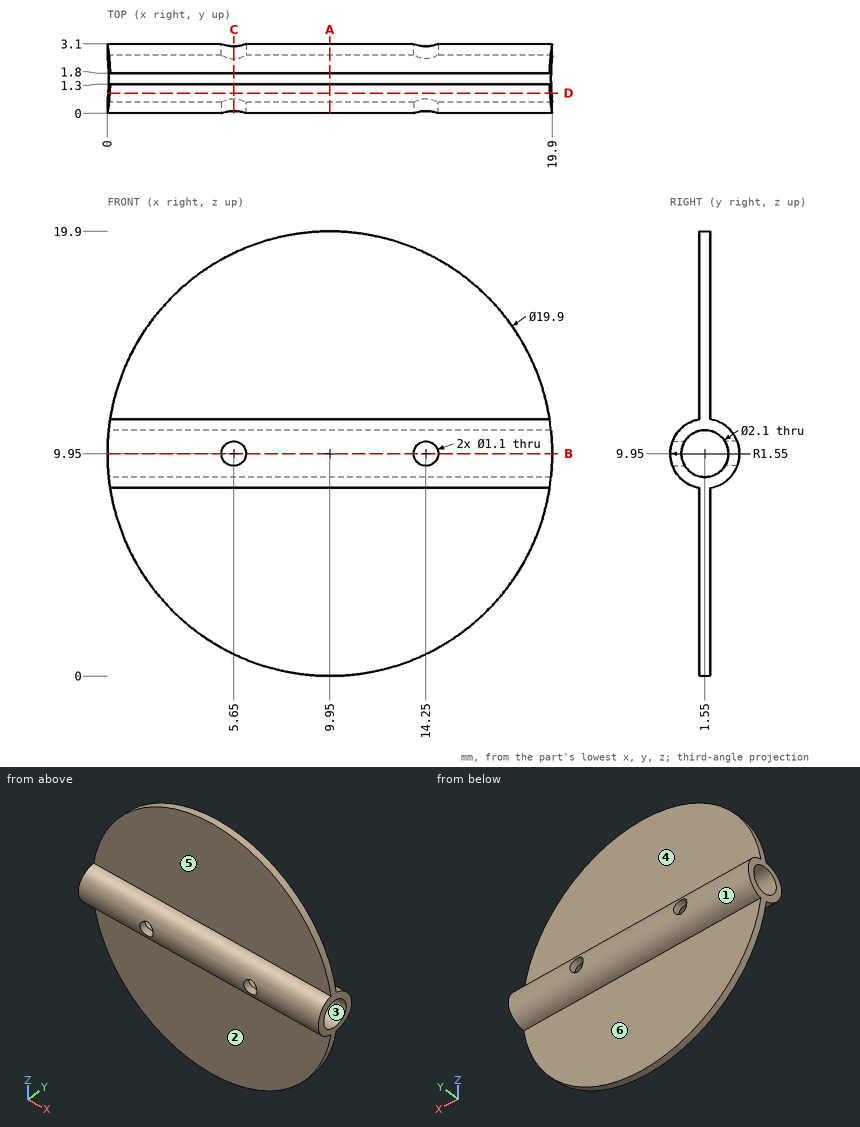
Here's the drawing with two shaded views (mm, measured from the low corner). I have some questions. A direction names the side the tool comes from. Coordinates: 2 decimals unless noted, no trailing zeros. Write each loop counter-clockwise with the first axis right and the second up, starting at its lowest first coordinate (ties: lowest second). Pieces come first, ordered by that corner, then holes. Notation, with made-up numbers: (81, 0) - (129, 0) arc R6 ccw to (129, 9) - close; hole circle Ø11 at (21.25, -17). An arc over 180 degrees is marked (long way). Return JSON: item names as keys, results as strings.
Q1. If we section it at A-A (x = 9.95): Please give me the cut outline in (y, z).
Computed values:
{"outline": "(1.3, 0) - (1.8, 0) - (1.8, 8.42) arc R1.55 ccw to (1.8, 11.48) - (1.8, 19.9) - (1.3, 19.9) - (1.3, 11.48) arc R1.55 ccw to (1.3, 8.42) - close; hole circle Ø2.1 at (1.55, 9.95)"}
Q2. If we section it at B-B (z = 9.95): Please give me the cut outline in (x, y).
Computed values:
{"outline": "(0, 0) - (5.1, 0) - (5.1, 0.5) - (0, 0.5) - close; (0, 2.6) - (5.1, 2.6) - (5.1, 3.1) - (0, 3.1) - close; (6.2, 0) - (13.7, 0) - (13.7, 0.5) - (6.2, 0.5) - close; (6.2, 2.6) - (13.7, 2.6) - (13.7, 3.1) - (6.2, 3.1) - close; (14.8, 0) - (19.9, 0) - (19.9, 0.5) - (14.8, 0.5) - close; (14.8, 2.6) - (19.9, 2.6) - (19.9, 3.1) - (14.8, 3.1) - close"}
Q3. On a 3-axis mill with a long thin cutter (end or side, diameter ignored), from which of +Z, -Z, +X, -X, +Y, -Y can I reach the whole of each face in a straight line? I mean the marked faces 4, 5 and 6. Say none if no direction works.
Computed values:
{"face 4": "+Z, +X, -X, +Y", "face 5": "+Z, +X, -X, -Y", "face 6": "-Z, +X, -X, +Y"}
Q4. Thinking about a two-plate mould opening in Y: for the marked faces 1, 2 and 3, which applies, +Y half, -Y half, draft (parallel to the pull), parting line (faces both ways), or undercut?
Computed values:
{"face 1": "+Y half", "face 2": "-Y half", "face 3": "undercut"}
Q5. If we section it at D-D (y = 0.9): Please give me the cut outline in (x, z).
Computed values:
{"outline": "(0.03, 9.13) arc R9.95 ccw to (0.1, 8.54) - (19.8, 8.54) arc R9.95 ccw to (19.87, 9.13) - close; (0.03, 10.77) - (19.87, 10.77) arc R9.95 ccw to (19.8, 11.36) - (0.1, 11.36) arc R9.95 ccw to start"}
Q6. Please list where these lines run through material, in increasing order: L1, parallel to Y at x = 4.5, z = 15.75; L2, parallel to Z at x = 12, y = 0.85; L3, parallel to Z at x = 4.25, y = 1.9. Write a range as from..to.
Computed values:
{"L1": "y = 1.3..1.8", "L2": "z = 8.57..9.17, 10.73..11.33", "L3": "z = 8.44..8.96, 10.94..11.46"}
Q7. I'm going to push flat-ended pins straight in: pin 1 Ø4 at (x, z) = (10, 4.5) entering from -Y; pin 2 Ø4 at (x, z) = (12, 4.5) entering from +Y; pin 3 Ø6 at (x, z) = (5, 6) entering from -Y. Where does each tip first touch, or does it pass through?
Computed values:
{"pin 1": "stops at y = 1.3", "pin 2": "stops at y = 1.8", "pin 3": "stops at y = 0.33"}
Q8. If we section it at C-C (x = 5.65): Please give me the cut outline in (y, z).
Computed values:
{"outline": "(0.1, 9.4) arc R1.55 ccw to (1.3, 8.42) - (1.3, 0.98) - (1.8, 0.98) - (1.8, 8.42) arc R1.55 ccw to (3, 9.4) - (2.44, 9.4) arc R1.05 cw to (0.66, 9.4) - close; (0.1, 10.5) - (0.66, 10.5) arc R1.05 cw to (2.44, 10.5) - (3, 10.5) arc R1.55 ccw to (1.8, 11.48) - (1.8, 18.92) - (1.3, 18.92) - (1.3, 11.48) arc R1.55 ccw to start"}
